Autodesk Inventor part; units mm, degrees
ref_plane "XZ Plane" through (0, 0, 0) normal (0, 1, 0) x (-1, 0, 0)
sketch "Sketch1" plane through (0, 0, 0) normal (0, 1, 0) x (-1, 0, 0)
  circle A0 centre (0, 0) radius 6.1
  circle A1 centre (0, 0) radius 4.9
  circle A2 centre (0, 0) radius 8.1
  circle A3 centre (0, 0) radius 2.9
  dimension "d0" = 12.2
  dimension "d1" = 9.8
  dimension "d2" = 2
  dimension "d5" = 2
extrude "Extrusion1" add sketch "Sketch1" along normal blind 3 contours A0 | A1 | A2 | A3
extrude "Extrusion2" add sketch "Sketch1" along normal blind 10
sketch "Sketch7" plane through (0, 0, 0) normal (0, -1, 0) x (1, 0, 0)
  circle A0 centre (0, 0) radius 8.1
  line L0 (7.7363, -2.4) -> (-7.7363, -2.4)
  line L1 (-7.7363, -2.4) -> (-7.7363, -5.4)
  line L2 (-7.7363, -5.4) -> (7.7363, -5.4)
  line L3 (7.7363, -5.4) -> (7.7363, -2.4)
  line L4 (7.7363, 2.4) -> (-7.7363, 2.4)
  line L5 (-7.7363, 2.4) -> (-7.7363, 5.4)
  line L6 (-7.7363, 5.4) -> (7.7363, 5.4)
  line L7 (7.7363, 5.4) -> (7.7363, 2.4)
  point P0 (6.0374, 5.4)
  point P1 (-6.0374, 5.4)
  point P2 (-6.0374, -5.4)
  point P3 (6.0374, -5.4)
  dimension "d34" = 3
  dimension "d35" = 3
  dimension "d36" = 4.8
  dimension "d37" = 2.4
extrude "Extrusion7" add sketch "Sketch7" along normal blind 7 contours L4 A0 L6 | A0 L2 L0
sketch "Sketch8" plane through (-6.0374, 0, 5.4) normal (0, 0, 1) x (1, 0, 0)
  circle A0 centre (3.0874, -3) radius 1.05
  circle A1 centre (8.9874, -3) radius 1.05
  line L0 (12.0748, 0) -> (0, 0)
  point P0 (6.0374, 0)
  dimension "d40" = 2.1
  dimension "d41" = 2.1
  dimension "d42" = 3
  dimension "d43" = 3
  dimension "d44" = 5.9
  dimension "d45" = 2.95
extrude "Extrusion8" cut sketch "Sketch8" against normal blind 20
sketch "Sketch9" plane through (0, 10, 0) normal (0, 1, 0) x (1, 0, 0)
  circle A0 centre (0, 0) radius 6.1
  circle A1 centre (0, 0) radius 2.9
  circle A2 centre (0, 0) radius 4.9
  circle A3 centre (0, 0) radius 8.1
extrude "Extrusion9" add sketch "Sketch9" along normal blind 2 contours A2
properties part number "Feather_0_clip"
Could you check a few things on this model? Use its own coordinates, in mm. A direction names the side the tool comes from. Give positions to 0.01 mm unless a question says otherwise; leave off trailing zeros. Loops run counter-clockwise (first coordinate to the right, second up) from the corner with the lowest first, then second, coordinate; pieces in that order, holes last. Notation, with made-up numbers: (-35, 1) - (-30, 1) arc R30 cw to (-30, 26) - close; hole circle Ø11 at (3, 29). An arc over 180 degrees is marked (long way). Use one line per item in the form item = value.
1. I want a section at C-C (z = 4). Please give me the cut outline in (x, y).
Response values:
outline = (-7.04, -7) - (7.04, -7) - (7.04, 10) - (4.61, 10) - (4.61, 3) - (2.83, 3) - (2.83, 12) - (-2.83, 12) - (-2.83, 3) - (-4.61, 3) - (-4.61, 10) - (-7.04, 10) - close; hole circle Ø2.1 at (-2.95, -3); hole circle Ø2.1 at (2.95, -3)
2. I need wall thicknesses on probe 1 along X at (y, z) = (5, 0); probe 2 along Z at (x, y) = (-2.5, -4.25); probe 3 along X at (y, z) = (-2.5, 5.25). Which ranges of each line are inside material? Lowest first, please.
Response values:
probe_1 = -8.1 to -6.1, -4.9 to -2.9, 2.9 to 4.9, 6.1 to 8.1
probe_2 = -5.4 to -2.4, 2.4 to 5.4
probe_3 = -6.17 to -3.87, -2.03 to 2.03, 3.87 to 6.17
3. On a 3-axis mill with a long thin cutter (end or side, diameter ignored), from which of +Z, -Z, +X, -X, +Y, -Y can I reach the whole of each face in a straight line? I mean faces 5 (the face through (-0.1, 12, 3.2)), 6 (the face through (0, 3, 0)), 7 (the face through (0, -3, 5.4)), 8 (the face through (0, -3, -5.4)), 9 (the face through (0, 0, 0)). Say none if no direction works.
Response values:
face_5 = +Z, -Z, +X, -X, +Y
face_6 = +Y
face_7 = +Z, +X, -X, -Y
face_8 = -Z, +X, -X, -Y
face_9 = +X, -X, -Y
4. I want a section at A-A (y = 7.5). Please give me the cut outline in (x, z).
Response values:
outline = circle Ø16.2 at (0, 0); circle Ø9.8 at (0, 0); hole circle Ø12.2 at (0, 0); hole circle Ø5.8 at (0, 0)
5. I'm going to push flat-ended pins straight in: pin 1 Ø2 at (x, y) = (-1.5, -2.5) entering from +Z; pin 2 Ø7.5 at (x, y) = (-1.5, -4) entering from -Z; pin 3 Ø8 at (y, z) = (9.5, -1.5) entering from -X; pin 4 Ø0.8 at (x, z) = (-3, 7) entering from -Y. Where does each tip first touch, or does it pass through?
Response values:
pin_1 = 5.4
pin_2 = -5.4
pin_3 = -8.1
pin_4 = 0
6. I want a section at D-D (x = 0). Please give me the cut outline in (y, z).
Response values:
outline = (-7, -5.4) - (0, -5.4) - (0, -8.1) - (10, -8.1) - (10, -6.1) - (3, -6.1) - (3, -4.9) - (12, -4.9) - (12, -2.9) - (3, -2.9) - (3, 2.9) - (12, 2.9) - (12, 4.9) - (3, 4.9) - (3, 6.1) - (10, 6.1) - (10, 8.1) - (0, 8.1) - (0, 5.4) - (-7, 5.4) - (-7, 2.4) - (0, 2.4) - (0, -2.4) - (-7, -2.4) - close
7. Thinking about a two-plate mould opening in Y: for faces 1 (the face through (-1.98, -3.4, -3.88)), 2 (the face through (0, -7, 4)), 3 (the face through (-1, 3, 5)), 4 (the face through (1.9, -3, 3.9)), which applies, released by +Y, released by -Y, zero draft, split by the parting line, or undercut?
Response values:
face_1 = undercut
face_2 = released by -Y
face_3 = released by +Y
face_4 = undercut
8. I want a section at B-B (y = -5.75). Please give me the cut outline in (x, z), and give its area (3 significant figures).
Response values:
outline = (-7.74, -2.4) arc R8.1 ccw to (-6.04, -5.4) - (6.04, -5.4) arc R8.1 ccw to (7.74, -2.4) - close; (-7.74, 2.4) - (7.74, 2.4) arc R8.1 ccw to (6.04, 5.4) - (-6.04, 5.4) arc R8.1 ccw to start
area = 84.4 mm²
